Part model, mm, in its own coordinate system. A direction names the side the tool comes from. Round coordinates to 2 decimals unless told otherwise and drop trailing zeros. Loops run counter-clockwise (first coordinate to the right, second up) from the corner with the lowest first, then second, coordinate; pieces in that order, holes last. Notation, with made-up numbers: M -2.5,-4.5 L 39.5,-4.5 A27 cw 39.5,16.5 Z; hole C 23,72 d5. An arc over 180 degrees is marked long. Put each result on its own line as item: value. Start each with the question number.
1) Drop flat-ended pins along their axis: pin 1 Ø1 at (x, z) = (2.5, 4) entering from -Y; pin 2 Ø4 at (y, z) = (-28, -3.5) entering from +X; pin 3 Ø5 at (x, y) = (4, -8.5) entering from -Z; pin 4 Ø4 at (x, z) = (1, 3.5) entering from +Y. Give the stop position or say it passes through.
2) Slice it at A-A on y = -6. Give the cut face in (x, z), then the cut area to 3 significant figures.
3) Pull direction Y, two halves, no side cores. Call faces 1 (the cylindrical face through (0.03, -3.14, 0.9)), 2 (the flat face through (2, -5, 3)), 3 (the flat face through (-3, -12, 0)): +Y half, -Y half, draft (parallel to the pull), parting line (faces both ways), or undercut.
4) Slice it at D-D on x = 4.25. Give the cut face in (y, z), then the cut area to 3 significant figures.
5) Which spindle directions (+Z, -Z, +X, -X, +Y, -Y) get a long thin tool onto all of the face, cutting with end or side? Do faces 4 (the flat face through (0, 0, 0)), 5 (the flat face through (-2, -5, -3)), 6 (the flat face through (3, -12, 0)). Say none if no direction does.
6) Slice it at C-C on y = -35. Give the cut face in (x, z).
7) Slice it at B-B on z = 2.25. Give the cut face in (x, y).
8) Probe line 1 along Z through (x, y) = (0.1, -6); line 2 along Z through (x, y) = (-0.8, -6); line 3 along Z through (x, y) = (-0.25, -56). List the from-to ranges inside material, lowest first.
```python
from build123d import *

# Parameters (mm, degrees)
F1_DEPTH = 70
F2_DEPTH = 12
F3_R     = 3
F4_DEPTH = 25
F5_R     = 5


with BuildPart() as f1:
    # F0 (on Front) → F1 (new body)
    with BuildSketch(Plane.XZ):
        with BuildLine():
            ThreePointArc((2, -4.582575695), (4.1833001327, -2.7386127875), (5, 0))
            ThreePointArc((5, 0), (4.1833001327, 2.7386127875), (2, 4.582575695))
            Line((2, 4.582575695), (2, -4.582575695))
        make_face()
        with BuildLine():
            Line((2, -4.582575695), (2, 4.582575695))
            ThreePointArc((2, 4.582575695), (0, 5), (-2, 4.582575695))
            Line((-2, 4.582575695), (-2, -4.582575695))
            ThreePointArc((-2, -4.582575695), (0, -5), (2, -4.582575695))
        make_face()
        with BuildLine():
            Line((-2, -4.582575695), (-2, 4.582575695))
            ThreePointArc((-2, 4.582575695), (-5, 0), (-2, -4.582575695))
        make_face()
    extrude(amount=F1_DEPTH)

    # F0 (on Front) → F2 (cut)
    with BuildSketch(Plane.XZ):
        with BuildLine():
            Line((-2, -4.582575695), (-2, 4.582575695))
            ThreePointArc((-2, 4.582575695), (-5, 0), (-2, -4.582575695))
        make_face()
        with BuildLine():
            ThreePointArc((2, -4.582575695), (4.1833001327, -2.7386127875), (5, 0))
            ThreePointArc((5, 0), (4.1833001327, 2.7386127875), (2, 4.582575695))
            Line((2, 4.582575695), (2, -4.582575695))
        make_face()
    extrude(amount=F2_DEPTH, mode=Mode.SUBTRACT)

    # F3 (on face) → F4 (cut)
    with BuildSketch(Plane.YZ.offset(2)):
        with Locations((-6, 0)):
            Circle(F3_R)
    extrude(amount=-F4_DEPTH, mode=Mode.SUBTRACT)

    # F5
    f5_edges = [f1.edges().sort_by_distance(p)[0] for p in [
        (2, -70, -4.582576),
    ]]
    fillet(f5_edges, radius=F5_R)


solid = f1.part
```
Recorded:
1. pin 1: stops at y = -67.69
1. pin 2: stops at x = 4.77
1. pin 3: stops at z = -4.77
1. pin 4: stops at y = 0
2. outline: M -2,-4.58 A5 ccw 2,-4.58 L 2,-3 L -2,-3 Z; M -2,3 L 2,3 L 2,4.58 A5 ccw -2,4.58 Z
2. area: 14.9 mm2
3. face 1: undercut
3. face 2: draft
3. face 3: +Y half
4. outline: M -65,-2.63 L -12,-2.63 L -12,2.63 L -65,2.63 A2.63 ccw Z
4. area: 290 mm2
5. face 4: +Z, -Z, +X, -X, +Y
5. face 5: +Z, -Z, -X, +Y
5. face 6: +Z, -Z, +X, +Y
6. outline: C 0,0 d10
7. outline: M -4.47,-65 A4.47 ccw 4.47,-65 L 4.47,-12 L 2,-12 L 2,-7.98 L -2,-7.98 L -2,-12 L -4.47,-12 Z; M -2,-4.02 L 2,-4.02 L 2,0 L -2,0 Z
8. line 1: z = -5 to -3, 3 to 5
8. line 2: z = -4.94 to -3, 3 to 4.94
8. line 3: z = -4.99 to 4.99
